Check sheet for the modelled part. Datum: model origin and axes. Units: mm. A direction names the side the tool comes from. Give positions to 0.01 mm unless a question says otherwise; leave off trailing zeros. Loops run counter-clockwise (first coordinate to the right, second up) from the corner with the lowest first, then second, coordinate; pieces in that order, holes last. Notation, with made-up numbers: M 89,48 L 111,48 A15 cw 111,66 Z; hole C 30.5,68.5 d3. An arc over 180 degrees is marked long. Write each question's results on one line, items separated by ' | '. Start each with the question number.
1. Tool access check on faces 4 (the flat face through (-20, 2, 6)), 5 (the flat face through (-15.3, 29, 13.4)), 6 (the cylindrical face through (0.1, 2, 34.5)). Record the directions out of +Z, -Z, +X, -X, +Y, -Y that give a thin tool (end or side, any length) a straight path to the whole face; none if there is none.
2. Sectioned sample at C-C on z = -13. Record the cut outline in (x, y), and give its area (3 significant figures).
3. Draft check along Z on faces 1 (the cylindrical face through (1.32, 0.99, -29.97)), 2 (the flat face through (-28.4, 0, -10.3)), 3 (the cylindrical face through (1.32, 23.72, -29.97)). Enter one of: pulls with the +Z half, pulls with the -Z half, needs draft (parallel to the pull), parting line crosses it, or undercut.
4. Go/stop test with flat-tipped pins: pin 1 (9.5 mm diameter, centred on x = 0, z = 37.5, fed in from +Y); pin 2 (8 mm diameter, centred on y = 32.5, z = 8, fed in from -X); pin 3 (3 mm diameter, centred on x = -15, y = 23.5, fed in from +Z); pin 4 (18 mm diameter, centred on x = 2, z = 7.5, fed in from -Y). Record where each tip stops, or that it passes through.
5. Sectioned sample at D-D on y = 40.5. Record the cut outline in (x, z).
6. Sectioned sample at A-A on z = 0. Record the cut outline in (x, y), and give its area (3 significant figures).
7. Material ranges on line 1 along X through (y, z) = (1, 0); line 2 along Z through (x, y) = (1, 33); line 3 along X through (y, z) = (41, 0), recorded low to high.
8. Sectioned sample at B-B on x = -37.5. Record the cut outline in (y, z).
```python
from build123d import *

# Parameters (mm, degrees)
CROQUIS1_R              = 43.5
CROQUIS1_R_2            = 30
SALIENTE_EXTRUIR1_DEPTH = 4
CROQUIS2_R              = 30
CROQUIS2_R_2            = 20
SALIENTE_EXTRUIR2_DEPTH = 44
CROQUIS3_R              = 30
CROQUIS3_R_2            = 20
CORTAR_EXTRUIR1_DEPTH   = 2
CROQUIS4_R              = 26
CORTAR_EXTRUIR2_DEPTH   = 15
CROQUIS5_R              = 3
CORTAR_EXTRUIR3_DEPTH   = 4


with BuildPart() as part:
    # Croquis1 → Saliente-Extruir1 (new body)
    with BuildSketch(Plane(origin=(0, 0, 0), x_dir=(1, 0, 0), z_dir=(0, 1, 0))):
        with Locations(Location((0, 0, 0), (0, 0, 270))):
            Circle(CROQUIS1_R)
        with Locations(Location((0, 0, 0), (0, 0, 270))):
            Circle(CROQUIS1_R_2, mode=Mode.SUBTRACT)
    extrude(amount=SALIENTE_EXTRUIR1_DEPTH)

    # Croquis2 → Saliente-Extruir2 (add)
    with BuildSketch(Plane(origin=(0, 0, 0), x_dir=(1, 0, 0), z_dir=(0, 1, 0))):
        with Locations(Location((0, 0, 0), (0, 0, 270))):
            Circle(CROQUIS2_R)
        with Locations(Location((0, 0, 0), (0, 0, 270))):
            Circle(CROQUIS2_R_2, mode=Mode.SUBTRACT)
    extrude(amount=SALIENTE_EXTRUIR2_DEPTH)

    # Croquis3 → Cortar-Extruir1 (cut)
    with BuildSketch(Plane(origin=(0, 0, 0), x_dir=(1, 0, 0), z_dir=(0, 1, 0))):
        with Locations(Location((0, 0, 0), (0, 0, 270))):
            Circle(CROQUIS3_R)
        with Locations(Location((0, 0, 0), (0, 0, 270))):
            Circle(CROQUIS3_R_2, mode=Mode.SUBTRACT)
    extrude(amount=CORTAR_EXTRUIR1_DEPTH, mode=Mode.SUBTRACT)

    # Croquis4 → Cortar-Extruir2 (cut)
    with BuildSketch(Plane(origin=(0, 44, 0), x_dir=(1, 0, 0), z_dir=(0, 1, 0))):
        with Locations(Location((0, 0, 0), (0, 0, 270))):
            Circle(CROQUIS4_R)
    extrude(amount=-CORTAR_EXTRUIR2_DEPTH, mode=Mode.SUBTRACT)

    # Croquis5 → Cortar-Extruir3 (cut)
    with BuildSketch(Plane(origin=(0, 0, 0), x_dir=(1, 0, 0), z_dir=(0, 1, 0))):
        with Locations(Location((0, -37.5, 0), (0, 0, 270))):
            Circle(CROQUIS5_R)
        with Locations(Location((-37.5, 0, 0), (0, 0, 270))):
            Circle(CROQUIS5_R)
        with Locations(Location((0, 37.5, 0), (0, 0, 270))):
            Circle(CROQUIS5_R)
        with Locations(Location((37.5, 0, 0), (0, 0, 270))):
            Circle(CROQUIS5_R)
    extrude(amount=CORTAR_EXTRUIR3_DEPTH, mode=Mode.SUBTRACT)


solid = part.part
```
Output values:
1) face 4: -Y | face 5: +Y | face 6: +Y, -Y
2) outline: M -41.51,0 L -27.04,0 L -27.04,2 L -15.2,2 L -15.2,29 L -22.52,29 L -22.52,44 L -27.04,44 L -27.04,4 L -41.51,4 Z; M 15.2,2 L 27.04,2 L 27.04,0 L 41.51,0 L 41.51,4 L 27.04,4 L 27.04,44 L 22.52,44 L 22.52,29 L 15.2,29 Z | area: 891 mm2
3) face 1: undercut | face 2: needs draft | face 3: parting line crosses it
4) pin 1: y = 4 | pin 2: x = -29.73 | pin 3: z = 26.79 | pin 4: through
5) outline: C 0,0 d60; hole C 0,0 d52
6) outline: M -43.5,0 L -40.5,0 L -40.5,4 L -43.5,4 Z; M -34.5,0 L -30,0 L -30,2 L -20,2 L -20,29 L -26,29 L -26,44 L -30,44 L -30,4 L -34.5,4 Z; M 20,2 L 30,2 L 30,0 L 34.5,0 L 34.5,4 L 30,4 L 30,44 L 26,44 L 26,29 L 20,29 Z; M 40.5,0 L 43.5,0 L 43.5,4 L 40.5,4 Z | area: 720 mm2
7) line 1: -43.5 to -40.5, -34.5 to -30, 30 to 34.5, 40.5 to 43.5 | line 2: -29.98 to -25.98, 25.98 to 29.98 | line 3: -30 to -26, 26 to 30
8) outline: M 0,-22.05 L 4,-22.05 L 4,-3 L 0,-3 Z; M 0,3 L 4,3 L 4,22.05 L 0,22.05 Z
